Model file for the job. Use its own axes, mm. A direction names the side the tool comes from. Coordinates: 2 decimals unless noted, no trailing zeros. Order: outer loops, then holes, each group sorted by start corner. A loop starts at its lowest first (then second) coordinate and runs counter-clockwise, first axis right, second up. Notation, with made-up numbers: M 6.25,-23.75 L 39.25,-23.75 A18 cw 39.25,-11.75 Z; hole C 15.5,-7 d2. An arc over 180 degrees is marked long. Return JSON: item names as keys, results as strings.
```python
from build123d import *

# Parameters (mm, degrees)
SKETCH1_W           = 260
SKETCH1_H           = 266
BOSS_EXTRUDE1_DEPTH = 6
SKETCH2_W           = 31.75
SKETCH2_H           = 6
SKETCH2_W_2         = 6
SKETCH2_H_2         = 25.4
TAB_CUT_OUTS_DEPTH  = 6
SKETCH4_W           = 12.7762
SKETCH4_H           = 3.2512
SKETCH4_W_2         = 3.2512
SKETCH4_H_2         = 12.7762
CUT_EXTRUDE1_DEPTH  = 7


with BuildPart() as part:
    # Sketch1 → Boss-Extrude1 (new body)
    with BuildSketch(Plane(origin=(0, 0, 0), x_dir=(1, 0, 0), z_dir=(0, 1, 0))):
        Rectangle(SKETCH1_W, SKETCH1_H)
    extrude(amount=BOSS_EXTRUDE1_DEPTH)

    # Sketch2 → Tab Cut Outs (cut)
    with BuildSketch(Plane(origin=(0, 6, 0), x_dir=(1, 0, 0), z_dir=(0, 1, 0))):
        with Locations((95.25, 130)):
            Rectangle(SKETCH2_W, SKETCH2_H)
        with Locations((-31.75, 130)):
            Rectangle(SKETCH2_W, SKETCH2_H)
        with Locations((-95.25, 130)):
            Rectangle(SKETCH2_W, SKETCH2_H)
        with Locations((31.75, 130)):
            Rectangle(SKETCH2_W, SKETCH2_H)
        with Locations((31.75, -130)):
            Rectangle(SKETCH2_W, SKETCH2_H)
        with Locations((95.25, -130)):
            Rectangle(SKETCH2_W, SKETCH2_H)
        with Locations((-95.25, -130)):
            Rectangle(SKETCH2_W, SKETCH2_H)
        with Locations((-31.75, -130)):
            Rectangle(SKETCH2_W, SKETCH2_H)
        with Locations((127, -95.25)):
            Rectangle(SKETCH2_W_2, SKETCH2_H_2)
        with Locations((127, 31.75)):
            Rectangle(SKETCH2_W_2, SKETCH2_H_2)
        with Locations((127, 95.25)):
            Rectangle(SKETCH2_W_2, SKETCH2_H_2)
        with Locations((127, -31.75)):
            Rectangle(SKETCH2_W_2, SKETCH2_H_2)
    extrude(amount=-TAB_CUT_OUTS_DEPTH, mode=Mode.SUBTRACT)

    # Sketch4 → Cut-Extrude1 (cut, through all)
    with BuildSketch(Plane(origin=(0, 6, 0), x_dir=(1, 0, 0), z_dir=(0, 1, 0))):
        with Locations((-64.9125, 102.6668)):
            Rectangle(SKETCH4_W, SKETCH4_H)
        with Locations((-102.9744, 88.3031)):
            Rectangle(SKETCH4_W_2, SKETCH4_H_2)
        with Locations((-102.9744, 110.7313)):
            Rectangle(SKETCH4_W_2, SKETCH4_H_2)
        with Locations((-52.1744, 110.7313)):
            Rectangle(SKETCH4_W_2, SKETCH4_H_2)
        with Locations((-115.7125, 102.6668)):
            Rectangle(SKETCH4_W, SKETCH4_H)
        with Locations((-90.2363, 102.479993419)):
            Rectangle(SKETCH4_W, SKETCH4_H)
        with Locations((-39.4363, 102.479993419)):
            Rectangle(SKETCH4_W, SKETCH4_H)
        with Locations((-52.1744, 88.3031)):
            Rectangle(SKETCH4_W_2, SKETCH4_H_2)
        with Locations((-14.1125, 102.6668)):
            Rectangle(SKETCH4_W, SKETCH4_H)
        with Locations((-1.3744, 110.7313)):
            Rectangle(SKETCH4_W_2, SKETCH4_H_2)
        with Locations((11.3637, 102.479993419)):
            Rectangle(SKETCH4_W, SKETCH4_H)
        with Locations((-1.3744, 88.3031)):
            Rectangle(SKETCH4_W_2, SKETCH4_H_2)
        with Locations((36.6875, 102.6668)):
            Rectangle(SKETCH4_W, SKETCH4_H)
        with Locations((49.4256, 110.7313)):
            Rectangle(SKETCH4_W_2, SKETCH4_H_2)
        with Locations((62.1637, 102.479993419)):
            Rectangle(SKETCH4_W, SKETCH4_H)
        with Locations((49.4256, 88.3031)):
            Rectangle(SKETCH4_W_2, SKETCH4_H_2)
        with Locations((87.4875, 102.6668)):
            Rectangle(SKETCH4_W, SKETCH4_H)
        with Locations((100.2256, 110.7313)):
            Rectangle(SKETCH4_W_2, SKETCH4_H_2)
        with Locations((112.9637, 102.479993419)):
            Rectangle(SKETCH4_W, SKETCH4_H)
        with Locations((100.2256, 88.3031)):
            Rectangle(SKETCH4_W_2, SKETCH4_H_2)
        with Locations((-52.1744, -88.3031)):
            Rectangle(SKETCH4_W_2, SKETCH4_H_2)
        with Locations((-39.4363, -102.479993419)):
            Rectangle(SKETCH4_W, SKETCH4_H)
        with Locations((-52.1744, -110.7313)):
            Rectangle(SKETCH4_W_2, SKETCH4_H_2)
        with Locations((-64.9125, -102.6668)):
            Rectangle(SKETCH4_W, SKETCH4_H)
        with Locations((-1.3744, -88.3031)):
            Rectangle(SKETCH4_W_2, SKETCH4_H_2)
        with Locations((11.3637, -102.479993419)):
            Rectangle(SKETCH4_W, SKETCH4_H)
        with Locations((-1.3744, -110.7313)):
            Rectangle(SKETCH4_W_2, SKETCH4_H_2)
        with Locations((-14.1125, -102.6668)):
            Rectangle(SKETCH4_W, SKETCH4_H)
        with Locations((49.4256, -88.3031)):
            Rectangle(SKETCH4_W_2, SKETCH4_H_2)
        with Locations((62.1637, -102.479993419)):
            Rectangle(SKETCH4_W, SKETCH4_H)
        with Locations((49.4256, -110.7313)):
            Rectangle(SKETCH4_W_2, SKETCH4_H_2)
        with Locations((36.6875, -102.6668)):
            Rectangle(SKETCH4_W, SKETCH4_H)
        with Locations((112.9637, -102.479993419)):
            Rectangle(SKETCH4_W, SKETCH4_H)
        with Locations((100.2256, -88.3031)):
            Rectangle(SKETCH4_W_2, SKETCH4_H_2)
        with Locations((100.2256, -110.7313)):
            Rectangle(SKETCH4_W_2, SKETCH4_H_2)
        with Locations((87.4875, -102.6668)):
            Rectangle(SKETCH4_W, SKETCH4_H)
        with Locations((-102.9744, -88.3031)):
            Rectangle(SKETCH4_W_2, SKETCH4_H_2)
        with Locations((-90.2363, -102.479993419)):
            Rectangle(SKETCH4_W, SKETCH4_H)
        with Locations((-102.9744, -110.7313)):
            Rectangle(SKETCH4_W_2, SKETCH4_H_2)
        with Locations((-115.7125, -102.6668)):
            Rectangle(SKETCH4_W, SKETCH4_H)
    extrude(amount=-CUT_EXTRUDE1_DEPTH, mode=Mode.SUBTRACT)


solid = part.part
```
Item 1: Drop flat-ended pins along their axis: pin 1 Ø1 at (y, z) = (3, 102.5) entering from +X; pin 2 Ø3 at (x, y) = (30, 4) entering from -Z. Give the stop position or say it passes through.
Check result:
{"pin 1": "stops at x = 124", "pin 2": "stops at z = -127"}
Item 2: Saw through at A-A (z = -113). Write the cut outline in (x, y).
Check result:
{"outline": "M -130,0 L -104.6,0 L -104.6,6 L -130,6 Z; M -101.35,0 L -53.8,0 L -53.8,6 L -101.35,6 Z; M -50.55,0 L -3,0 L -3,6 L -50.55,6 Z; M 0.25,0 L 47.8,0 L 47.8,6 L 0.25,6 Z; M 51.05,0 L 98.6,0 L 98.6,6 L 51.05,6 Z; M 101.85,0 L 130,0 L 130,6 L 101.85,6 Z"}
Item 3: Saw through at C-C (z = 39). Write the cut outline in (x, y).
Check result:
{"outline": "M -130,0 L 124,0 L 124,6 L -130,6 Z"}
Item 4: 3-axis set-ups, long thin cutter, end or side, ignore diameter. For faces 1 (the flat face through (127, 3, 44.45)), 2 (the flat face through (79.375, 3, 130)), 3 (the flat face through (113, 3, 104.106)), 4 (the flat face through (130, 3, -63)), 5 (the flat face through (47.625, 3, -130)): which of +Z, -Z, +X, -X, +Y, -Y reach the whole face in a straight line?
Check result:
{"face 1": "+X, +Y, -Y", "face 2": "+Z, +Y, -Y", "face 3": "+Y, -Y", "face 4": "+Z, -Z, +X, +Y, -Y", "face 5": "-Z, +Y, -Y"}
Item 5: Wall check: line 1 (Z direction, x = -53.5, y = 3.45) (3 decimals); line 2 (Z direction, x = 34, y = 2.1); line 3 (X direction, y = 1.1, z = -116.5). Give the ranges that are in metal, low to high.
Check result:
{"line 1": "z = -133 to -117.119, -104.343 to -94.691, -81.915 to 81.915, 94.691 to 104.343, 117.119 to 133", "line 2": "z = -127 to -104.29, -101.04 to 101.04, 104.29 to 127", "line 3": "x = -130 to -104.6, -101.35 to -53.8, -50.55 to -3, 0.25 to 47.8, 51.05 to 98.6, 101.85 to 130"}
Item 6: Saw through at B-B (y = 4.4). Count the separate pieces of the cut face and the enclosed holes in it, and give its area (3 significant figures).
Check result:
{"separate pieces": "1", "enclosed holes": "40", "area": "65,400 mm2"}
